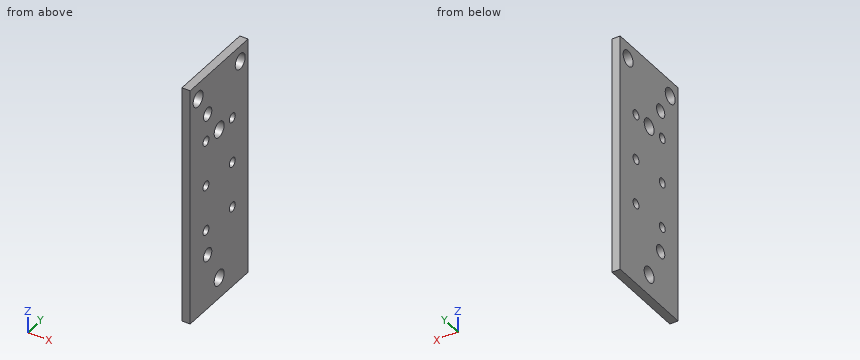
```python
from build123d import *

# Parameters (mm, degrees)
SKETCH1_W                      = 38.1
SKETCH1_H                      = 120
BOSS_EXTRUDE1_DEPTH            = 38.1
SKETCH2_W                      = 34.925
SKETCH2_H                      = 34.925
CUT_EXTRUDE1_DEPTH             = 130.767142413
F_4_2_4_2_DIAMETER_HOLE1_D     = 4.2
F_6_0_6_DIAMETER_HOLE1_D       = 6
F_4_2_4_2_DIAMETER_HOLE2_D     = 4.2
F_4_2_4_2_DIAMETER_HOLE2_DEPTH = 38.1
F_6_0_6_DIAMETER_HOLE2_D       = 6
F_6_0_6_DIAMETER_HOLE2_DEPTH   = 38.1
F_6_0_6_DIAMETER_HOLE3_D       = 6
F_6_0_6_DIAMETER_HOLE3_DEPTH   = 38.1
F_4_2_4_2_DIAMETER_HOLE3_D     = 4.2
SKETCH15_R                     = 2.1
SKETCH15_R_2                   = 3
BOSS_EXTRUDE2_DEPTH            = 3.175
BOSS_EXTRUDE3_START            = -3.175
SKETCH16_R                     = 2.1
BOSS_EXTRUDE3_DEPTH            = 3.175
SKETCH18_W                     = 3.175
SKETCH18_H                     = 3.175
CUT_EXTRUDE2_DEPTH             = 130.767142413
CUT_EXTRUDE3_START             = -3.175
CUT_EXTRUDE3_OUTLINE_R         = 2.1
CUT_EXTRUDE3_DEPTH             = 3.175
BOSS_EXTRUDE4_START            = -3.175
BOSS_EXTRUDE4_OUTLINE_R        = 3
BOSS_EXTRUDE4_DEPTH            = 3.175
SKETCH19_R                     = 3
CUT_EXTRUDE4_DEPTH             = 121.228267267
BOSS_EXTRUDE5_START            = -3.175
SKETCH20_R                     = 2.1
SKETCH20_R_2                   = 3
BOSS_EXTRUDE5_DEPTH            = 3.175
SKETCH23_R                     = 1.778
SKETCH23_R_2                   = 2.5
CUT_EXTRUDE5_DEPTH             = 121.228267267
SKETCH24_W                     = 5
SKETCH24_H                     = 34.925
CUT_EXTRUDE6_DEPTH             = 121.228267267
CUT_EXTRUDE7_DEPTH             = 121.228267267
CUT_EXTRUDE7_DEPTH_BACK        = 121.228267267
SKETCH25_W                     = 23.7
SKETCH25_H                     = 34.925


# Read off the part's stored shape, not the designer's step: Cut-Extrude3, Boss-Extrude4
with BuildPart() as part:
    # Sketch1 → Boss-Extrude1 (new body)
    with BuildSketch(Plane.XZ.offset(34.925)):
        with Locations((15.875, -55)):
            Rectangle(SKETCH1_W, SKETCH1_H)
    extrude(amount=-BOSS_EXTRUDE1_DEPTH)

    # Sketch2 → Cut-Extrude1 (cut, through all)
    with BuildSketch(Plane(origin=(0, 0, -115), x_dir=(-1, 0, 0), z_dir=(0, 0, -1))):
        with Locations((-17.4625, -17.4625)):
            Rectangle(SKETCH2_W, SKETCH2_H)
    extrude(amount=-CUT_EXTRUDE1_DEPTH, mode=Mode.SUBTRACT)

    # Ø4.2 (4.2) Diameter Hole1 (through all)
    with Locations(Plane(origin=(0, 0, 0), x_dir=(-1, 0, 0), z_dir=(0, -1, 0))):
        with Locations((-5, 35.97), (-5, 91.03)):
            Hole(F_4_2_4_2_DIAMETER_HOLE1_D / 2)

    # Ø6.0 (6) Diameter Hole1 (through all)
    with Locations(Plane(origin=(0, 0, 0), x_dir=(-1, 0, 0), z_dir=(0, -1, 0))):
        with Locations((-22.225, 106.5), (-22.225, 46.5)):
            Hole(F_6_0_6_DIAMETER_HOLE1_D / 2)

    # Ø4.2 (4.2) Diameter Hole2
    with Locations(Plane(origin=(0, 3.175, 0), x_dir=(1, 0, 0), z_dir=(0, 1, 0))):
        with Locations((22.225, 33.5), (22.225, 93.5), (29.296067812, 100.571067812), (29.296067812, 26.428932188)):
            Hole(F_4_2_4_2_DIAMETER_HOLE2_D / 2, depth=F_4_2_4_2_DIAMETER_HOLE2_DEPTH)

    # Ø6.0 (6) Diameter Hole2
    with Locations(Plane(origin=(0, 3.175, 0), x_dir=(1, 0, 0), z_dir=(0, 1, 0))):
        with Locations((24.925, 6)):
            Hole(F_6_0_6_DIAMETER_HOLE2_D / 2, depth=F_6_0_6_DIAMETER_HOLE2_DEPTH)

    # Ø6.0 (6) Diameter Hole3
    with Locations(Plane.ZY.offset(3.175)):
        with Locations((-6, -24.925), (-106.5, -22.225), (-46.5, -22.225)):
            Hole(F_6_0_6_DIAMETER_HOLE3_D / 2, depth=F_6_0_6_DIAMETER_HOLE3_DEPTH)

    # Ø4.2 (4.2) Diameter Hole3 (through all)
    with Locations(Plane.ZY.offset(3.175)):
        with Locations((-93.5, -22.225), (-33.5, -22.225), (-35.97, -5), (-91.03, -5), (-100.571067812, -29.296067812), (-26.428932188, -29.296067812)):
            Hole(F_4_2_4_2_DIAMETER_HOLE3_D / 2)

    # Sketch15 → Boss-Extrude2 (add)
    with BuildSketch(Plane(origin=(0, 3.175, 0), x_dir=(1, 0, 0), z_dir=(0, 1, 0))):
        with Locations((29.296067812, 26.428932188)):
            Circle(SKETCH15_R)
        with Locations((29.296067812, 100.571067812)):
            Circle(SKETCH15_R)
        with Locations((22.225, 106.5)):
            Circle(SKETCH15_R_2)
        with Locations((22.225, 46.5)):
            Circle(SKETCH15_R_2)
        with Locations((5, 35.97)):
            Circle(SKETCH15_R)
        with Locations((5, 91.03)):
            Circle(SKETCH15_R)
    extrude(amount=-BOSS_EXTRUDE2_DEPTH)

    # Sketch16 → Boss-Extrude3 (add)
    with BuildSketch(Plane.ZY.offset(3.175).offset(BOSS_EXTRUDE3_START)):
        with Locations((-100.571067812, -29.296067812)):
            Circle(SKETCH16_R)
        with Locations((-26.428932188, -29.296067812)):
            Circle(SKETCH16_R)
        with Locations((-35.97, -5)):
            Circle(SKETCH16_R)
        with Locations((-91.03, -5)):
            Circle(SKETCH16_R)
    extrude(amount=BOSS_EXTRUDE3_DEPTH)

    # Sketch18 → Cut-Extrude2 (cut, through all)
    with BuildSketch(Plane.XY.offset(5)):
        with Locations((-1.5875, 1.5875)):
            Rectangle(SKETCH18_W, SKETCH18_H)
    extrude(amount=-CUT_EXTRUDE2_DEPTH, mode=Mode.SUBTRACT)


with BuildPart() as body_2:
    # of the pieces the cut leaves, the one that is kept (cut_extrude2_keep)
    add(part.part.solids().sort_by_distance((-3.175, -34.925, -115))[0])

    # Cut-Extrude3 outline → Cut-Extrude3 (cut)
    with BuildSketch(Plane.YZ.offset(CUT_EXTRUDE3_START)):
        with Locations((-5, -91.03)):
            Circle(CUT_EXTRUDE3_OUTLINE_R)
        with Locations((-5, -35.97)):
            Circle(CUT_EXTRUDE3_OUTLINE_R)
        with Locations((-29.296067812, -26.428932188)):
            Circle(CUT_EXTRUDE3_OUTLINE_R)
        with Locations((-29.296067812, -100.571067812)):
            Circle(CUT_EXTRUDE3_OUTLINE_R)
    extrude(amount=CUT_EXTRUDE3_DEPTH, mode=Mode.SUBTRACT)

    # Boss-Extrude4 outline → Boss-Extrude4 (add)
    with BuildSketch(Plane.YZ.offset(BOSS_EXTRUDE4_START)):
        with Locations((-22.225, -46.5)):
            Circle(BOSS_EXTRUDE4_OUTLINE_R)
        with Locations((-22.225, -106.5)):
            Circle(BOSS_EXTRUDE4_OUTLINE_R)
        with Locations((-24.925, -6)):
            Circle(BOSS_EXTRUDE4_OUTLINE_R)
    extrude(amount=BOSS_EXTRUDE4_DEPTH)

    # Sketch19 → Cut-Extrude4 (cut, through all)
    with BuildSketch(Plane.ZY.offset(3.175)):
        with Locations((-6, -4.7625)):
            Circle(SKETCH19_R)
        with Locations((-6, -30.1625)):
            Circle(SKETCH19_R)
        with Locations((-25.3, -17.4625)):
            Circle(SKETCH19_R)
        with Locations((-83.29, -17.4625)):
            Circle(SKETCH19_R)
    extrude(amount=-CUT_EXTRUDE4_DEPTH, mode=Mode.SUBTRACT)

    # Sketch20 → Boss-Extrude5 (add)
    with BuildSketch(Plane(origin=(0, 0, 0), x_dir=(0, 0, -1), z_dir=(1, 0, 0)).offset(BOSS_EXTRUDE5_START)):
        with Locations((26.428932188, -29.296067812)):
            Circle(SKETCH20_R)
        with Locations((33.8, -17.4625)):
            Circle(SKETCH20_R_2)
        with Locations((33.5, -22.225)):
            Circle(SKETCH20_R)
        with Locations((35.97, -5)):
            Circle(SKETCH20_R)
        with Locations((91.03, -5)):
            Circle(SKETCH20_R)
        with Locations((93.8, -17.4625)):
            Circle(SKETCH20_R_2)
        with Locations((93.5, -22.225)):
            Circle(SKETCH20_R)
        with Locations((100.571067812, -29.296067812)):
            Circle(SKETCH20_R)
    extrude(amount=BOSS_EXTRUDE5_DEPTH)

    # Sketch23 → Cut-Extrude5 (cut, through all)
    with BuildSketch(Plane(origin=(0, 0, 0), x_dir=(0, 0, -1), z_dir=(1, 0, 0))):
        with Locations((42.75, -9.525)):
            Circle(SKETCH23_R)
        with Locations((25.3, -9.525)):
            Circle(SKETCH23_R)
        with Locations((15.22, -24.4)):
            Circle(SKETCH23_R_2)
        with Locations((25.3, -25.4)):
            Circle(SKETCH23_R)
        with Locations((42.75, -25.4)):
            Circle(SKETCH23_R)
        with Locations((60.2, -9.525)):
            Circle(SKETCH23_R)
        with Locations((60.2, -25.4)):
            Circle(SKETCH23_R)
        with Locations((70.28, -24.4)):
            Circle(SKETCH23_R_2)
    extrude(amount=-CUT_EXTRUDE5_DEPTH, mode=Mode.SUBTRACT)

    # Sketch24 → Cut-Extrude6 (cut, through all)
    with BuildSketch(Plane(origin=(0, 0, 0), x_dir=(0, 0, -1), z_dir=(1, 0, 0))):
        with Locations((-2.5, -17.4625)):
            Rectangle(SKETCH24_W, SKETCH24_H)
    extrude(amount=-CUT_EXTRUDE6_DEPTH, mode=Mode.SUBTRACT)

    # Sketch25 → Cut-Extrude7 (cut, two sides: drawn at the far end of the back side and taken through both)
    with BuildSketch(Plane(origin=(0, 0, 0), x_dir=(0, 0, -1), z_dir=(1, 0, 0)).offset(-CUT_EXTRUDE7_DEPTH_BACK)):
        with Locations((103.15, -17.4625)):
            Rectangle(SKETCH25_W, SKETCH25_H)
    extrude(amount=CUT_EXTRUDE7_DEPTH + CUT_EXTRUDE7_DEPTH_BACK, mode=Mode.SUBTRACT)


solid = body_2.part
```
Build history of the part. All positions in model axes, mm. Round coordinates to 2 decimals unless told otherwise and drop trailing zeros. Write each loop counter-clockwise with the first axis right and the second up, starting at its lowest first coordinate (ties: lowest second). Pieces come first, ordered by that corner, then holes.
1) Band-saw the part on A-A, the plane z = -60.2. List the corners of the cut face in (x, y) (3 decimals), and give its area (3 significant figures).
2) Band-saw the part on B-B, the plane z = -25.3. List the corners of the cut face in (x, y) (1 decimal).
3) Drill centre lines: probe 1 along Y at (x, z) = (-2.5, -60.2) (3 decimals); probe 2 along Y at (x, z) = (-2.35, -15.22) (3 decimals); probe 3 along Z at (x, y) = (-1.7, -24.5). Where is each one in solid material? Low to high.
4) Band-saw the part on C-C, the plane y = -31. List the corners of the cut face in (x, z) (3 decimals), and give its area (3 significant figures).
5) Band-saw the part on D-D, the plane z = -70.28. List the corners of the cut face in (x, y) (3 decimals).
Ans:
1. outline: (-3.175, -34.925) - (0, -34.925) - (0, -27.178) - (-3.175, -27.178) - close; (-3.175, -23.622) - (0, -23.622) - (0, -11.303) - (-3.175, -11.303) - close; (-3.175, -7.747) - (0, -7.747) - (0, 0) - (-3.175, 0) - close
1. area: 88.3 mm2
2. outline: (-3.2, -34.9) - (0, -34.9) - (0, -27.2) - (-3.2, -27.2) - close; (-3.2, -23.6) - (0, -23.6) - (0, -20.5) - (-3.2, -20.5) - close; (-3.2, -14.5) - (0, -14.5) - (0, -11.3) - (-3.2, -11.3) - close; (-3.2, -7.7) - (0, -7.7) - (0, 0) - (-3.2, 0) - close
3. probe 1: y = -34.925 to -27.178, -23.622 to -11.303, -7.747 to 0
3. probe 2: y = -34.925 to -26.9, -21.9 to 0
3. probe 3: z = -91.3 to -72.78, -67.78 to -61.73, -58.67 to -44.28, -41.22 to -26.83, -23.77 to -17.72, -12.72 to 0
4. outline: (-3.175, -91.3) - (0, -91.3) - (0, -8.881) - (-3.175, -8.881) - close; (-3.175, -3.119) - (0, -3.119) - (0, 0) - (-3.175, 0) - close
4. area: 272 mm2
5. outline: (-3.175, -34.925) - (0, -34.925) - (0, -26.9) - (-3.175, -26.9) - close; (-3.175, -21.9) - (0, -21.9) - (0, 0) - (-3.175, 0) - close
